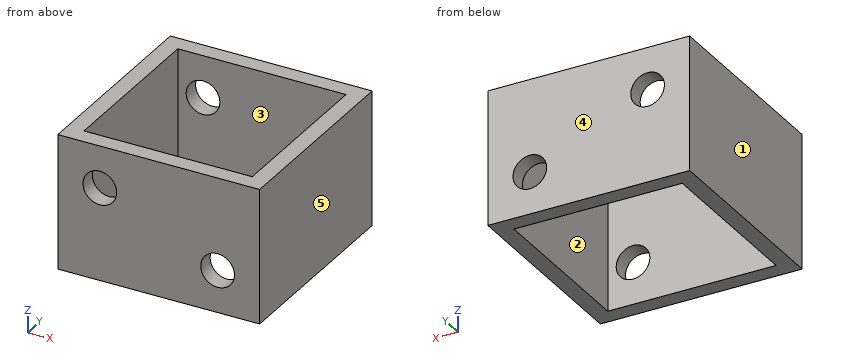
from build123d import *

# Parameters (mm, degrees)
SKETCH1_W           = 38.1
SKETCH1_H           = 38.1
SKETCH1_W_2         = 31.75
SKETCH1_H_2         = 31.75
BOSS_EXTRUDE1_DEPTH = 25.4
SKETCH2_R           = 3.175
CUT_EXTRUDE1_DEPTH  = 39.1


with BuildPart() as part:
    # Sketch1 → Boss-Extrude1 (new body)
    with BuildSketch(Plane.XY):
        with Locations((19.05, 19.05)):
            Rectangle(SKETCH1_W, SKETCH1_H)
        with Locations((19.05, 19.05)):
            Rectangle(SKETCH1_W_2, SKETCH1_H_2, mode=Mode.SUBTRACT)
    extrude(amount=BOSS_EXTRUDE1_DEPTH)

    # Sketch2 → Cut-Extrude1 (cut, through all)
    with BuildSketch(Plane.XZ):
        with Locations((7.9375, 17.4625)):
            Circle(SKETCH2_R)
        with Locations((30.1625, 7.9375)):
            Circle(SKETCH2_R)
    extrude(amount=-CUT_EXTRUDE1_DEPTH, mode=Mode.SUBTRACT)


solid = part.part
Geometry check sheet. Reference: the model listing, model coordinates, mm. Face numbers are marked on the shaded views. A direction names the side the tool comes from. Coordinates: 2 decimals unless noted, no trailing zeros. Loops run counter-clockwise (first coordinate to the right, second up) from the corner with the lowest first, then second, coordinate; pieces in that order, holes last. Notation, with made-up numbers: (61.25, 84) - (82.25, 84) arc R6 ccw to (82.25, 94) - close; hole circle Ø10 at (-39, -34.75). An arc over 180 degrees is marked (long way). Use one line per item in the form item = value. Start each with the question number.
Item 1: Section check D-D, the plane y = 36. Give the number of separate pieces and of enclosed holes in the cut face, and give its area (3 significant figures).
Item 2: Thickness scan on probe 1 along X at (y, z) = (14.5, 20) (3 decimals). Record the ranges inside material, lowest first.
Item 3: Gauge pin test, flat ends, axial feed: pin 1 (5 mm diameter, centred on x = 30.16, z = 7.94, fed in from +Y); pin 2 (7.5 mm diameter, centred on y = 24.5, z = 11.5, fed in from -X). Record the tip position at first contact, or that the pin passes through.
Item 4: Section check A-A, the plane y = 23.5. Enter the section's corners in (x, z) (3 decimals), and give its area (3 significant figures).
Item 5: Mould release check, pull along X, two halves, no side actions. Record for the marked faces 3, 4 and 5: +X half, -X half, draft (parallel to the pull), parting line (faces both ways), or undercut.
Item 6: Tool access check on the marked faces 1 and 2. Record the directions out of +Z, -Z, +X, -X, +Y, -Y that give a thin tool (end or side, any length) a straight path to the whole face; none if there is none.
Item 7: Section check C-C, the plane z = 21.25. Enter the section's corners in (x, y) (3 decimals).
Computed:
q1.separate_pieces = 1
q1.enclosed_holes = 2
q1.area = 904 mm2
q2.probe_1 = 0 to 3.175, 34.925 to 38.1
q3.pin_1 = through
q3.pin_2 = 0
q4.outline = (0, 0) - (3.175, 0) - (3.175, 25.4) - (0, 25.4) - close; (34.925, 0) - (38.1, 0) - (38.1, 25.4) - (34.925, 25.4) - close
q4.area = 161 mm2
q5.face_3 = undercut
q5.face_4 = draft
q5.face_5 = +X half
q6.face_1 = +Z, -Z, -X, +Y, -Y
q6.face_2 = +Z, -Z
q7.outline = (0, 0) - (38.1, 0) - (38.1, 38.1) - (0, 38.1) - close; hole (3.175, 3.175) - (34.925, 3.175) - (34.925, 34.925) - (3.175, 34.925) - close
